Source: CAD feature listing. Evaluate the final solid. Frame: model axes, mm. Give positions to 0.01 mm unless a question says otherwise; leave off trailing zeros. Order: outer loops, then holes, each group sorted by start corner. A loop starts at its lowest first (then second) coordinate and runs counter-clockwise, first axis right, second up. Notation, with made-up numbers: M 37,18 L 59,18 A12 ccw 59,38 Z; hole C -38.5,0 d8. An arc over 180 degrees is marked long. Return JSON: item names as keys, results as strings.
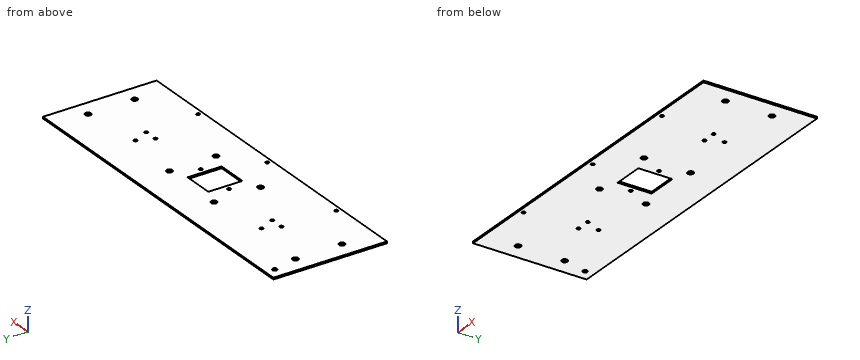
from build123d import *

# Parameters (mm, degrees)
F0_W     = 300
F0_H     = 100
F0_R     = 1.5
F0_R_2   = 2.55
F0_R_3   = 2
F0_W_2   = 27
F0_H_2   = 30
F1_DEPTH = 1.5


with BuildPart() as f1:
    # F0 (on Top) → F1 (new body)
    with BuildSketch(Plane.XY):
        with Locations((150, 50)):
            Rectangle(F0_W, F0_H)
        with Locations((60, 4)):
            Circle(F0_R, mode=Mode.SUBTRACT)
        with Locations((15, 29.5)):
            Circle(F0_R_2, mode=Mode.SUBTRACT)
        with Locations((121, 29.5)):
            Circle(F0_R_2, mode=Mode.SUBTRACT)
        with Locations((150, 4)):
            Circle(F0_R, mode=Mode.SUBTRACT)
        with Locations((240, 4)):
            Circle(F0_R, mode=Mode.SUBTRACT)
        with Locations((179, 29.5)):
            Circle(F0_R_2, mode=Mode.SUBTRACT)
        with Locations((285, 29.5)):
            Circle(F0_R_2, mode=Mode.SUBTRACT)
        with Locations((62, 51)):
            Circle(F0_R, mode=Mode.SUBTRACT)
        with Locations((74, 51)):
            Circle(F0_R, mode=Mode.SUBTRACT)
        with Locations((15, 70.5)):
            Circle(F0_R_2, mode=Mode.SUBTRACT)
        with Locations((68, 64.5)):
            Circle(F0_R, mode=Mode.SUBTRACT)
        with Locations((131.5, 50)):
            Circle(F0_R, mode=Mode.SUBTRACT)
        with Locations((121, 70.5)):
            Circle(F0_R_2, mode=Mode.SUBTRACT)
        with Locations((10, 92)):
            Circle(F0_R_3, mode=Mode.SUBTRACT)
        with Locations((150, 50)):
            Rectangle(F0_W_2, F0_H_2, mode=Mode.SUBTRACT)
        with Locations((168.5, 50)):
            Circle(F0_R, mode=Mode.SUBTRACT)
        with Locations((179, 70.5)):
            Circle(F0_R_2, mode=Mode.SUBTRACT)
        with Locations((226, 51)):
            Circle(F0_R, mode=Mode.SUBTRACT)
        with Locations((238, 51)):
            Circle(F0_R, mode=Mode.SUBTRACT)
        with Locations((232, 64.5)):
            Circle(F0_R, mode=Mode.SUBTRACT)
        with Locations((285, 70.5)):
            Circle(F0_R_2, mode=Mode.SUBTRACT)
    extrude(amount=-F1_DEPTH)


solid = f1.part
1. Ray query, probe 1 along Y at (x, z) = (150, -0.75); probe 2 along Y at (x, z) = (285, -0.9); probe 3 along Y at (x, z) = (240, -0.9). Return the intervals inside material, ascending.
Evaluation:
{"probe 1": "y = 0 to 2.5, 5.5 to 35, 65 to 100", "probe 2": "y = 0 to 26.95, 32.05 to 67.95, 73.05 to 100", "probe 3": "y = 0 to 2.5, 5.5 to 100"}
2. Section query B-B (x = 179). Return loops of the section in (y, z).
Evaluation:
{"outline": "M 0,-1.5 L 26.95,-1.5 L 26.95,0 L 0,0 Z; M 32.05,-1.5 L 67.95,-1.5 L 67.95,0 L 32.05,0 Z; M 73.05,-1.5 L 100,-1.5 L 100,0 L 73.05,0 Z"}
3. Section query C-C (y = 38). Return loops of the section in (x, z).
Evaluation:
{"outline": "M 0,-1.5 L 136.5,-1.5 L 136.5,0 L 0,0 Z; M 163.5,-1.5 L 300,-1.5 L 300,0 L 163.5,0 Z"}
4. Section query A-A (z = -0.3). State how many separate pieces and enclosed holes the cut face has, then the cut area to 3 significant figures.
Evaluation:
{"separate pieces": "1", "enclosed holes": "21", "area": "28,900 mm^2"}
